The listing builds one solid part. Answer for the finished solid, in the listing's coordinates (mm). A direction names the side the tool comes from. Coordinates: 2 decimals unless noted, no trailing zeros. Write each loop counter-clockwise with the first axis right and the second up, starting at its lowest first coordinate (ties: lowest second). Pieces come first, ordered by that corner, then holes. Notation, with made-up numbers: M -35,-2.5 L 18,-2.5 A15 cw 18,2.5 Z; hole C 33,36 d9. An arc over 180 degrees is marked long. Answer as CSV lines item,"result".
```python
from build123d import *

# Parameters (mm, degrees)
BOSS_EXTRUDE1_DEPTH = 3
SKETCH5_W           = 35
SKETCH5_H           = 23
BOSS_EXTRUDE2_DEPTH = 3
BOSS_EXTRUDE5_DEPTH = 35
BOSS_EXTRUDE8_START = -35
BOSS_EXTRUDE8_DEPTH = 35
CUT_EXTRUDE1_START  = -96
SKETCH11_R          = 2.9
CUT_EXTRUDE1_DEPTH  = 96
BOSS_EXTRUDE7_DEPTH = 1
SKETCH17_R          = 2.5
CUT_EXTRUDE2_DEPTH  = 10
SKETCH18_R          = 2
CUT_EXTRUDE3_DEPTH  = 10
SKETCH19_R          = 2
CUT_EXTRUDE4_DEPTH  = 4
SKETCH21_R          = 2
CUT_EXTRUDE5_DEPTH  = 7
SKETCH22_R          = 2.5
CUT_EXTRUDE6_DEPTH  = 4
FILLET1_R           = 10
FILLET2_R           = 2
FILLET3_R           = 2
FILLET4_R           = 1


with BuildPart() as part:
    # Sketch1 → Boss-Extrude1 (new body)
    with BuildSketch(Plane(origin=(0, 0, 0), x_dir=(1, 0, 0), z_dir=(0, 1, 0))):
        Polygon((0, 0), (0, 23), (8.5, 23), (8.5, 33), (17.5, 33), (17.5, 23), (26, 23), (26, 0), (61, 0), (61, 28.801365462), (61, 67.406151765), (50.5, 93.029580251), (50.5, 160), (-24.5, 160), (-24.5, 93.029580251), (-35, 67.406151765), (-35, 28.801365462), (-35, 0), align=None)
    extrude(amount=BOSS_EXTRUDE1_DEPTH)

    # Sketch5 → Boss-Extrude2 (add)
    with BuildSketch(Plane(origin=(0, 3, 0), x_dir=(1, 0, 0), z_dir=(0, 1, 0))):
        with Locations((-17.5, 11.5)):
            Rectangle(SKETCH5_W, SKETCH5_H)
        with Locations((43.5, 11.5)):
            Rectangle(SKETCH5_W, SKETCH5_H)
    extrude(amount=BOSS_EXTRUDE2_DEPTH)

    # Sketch12 → Boss-Extrude5 (add)
    with BuildSketch(Plane.ZY.offset(35)):
        with BuildLine():
            Line((-7.857598958, 0), (1.361945499, 0))
            ThreePointArc((1.361945499, 0), (-3.247826729, 8.5), (-7.857598958, 0))
        make_face()
    extrude(amount=-BOSS_EXTRUDE5_DEPTH)

    # Sketch15 → Boss-Extrude8 (add)
    with BuildSketch(Plane(origin=(61, 0, 0), x_dir=(0, 0, -1), z_dir=(1, 0, 0)).offset(BOSS_EXTRUDE8_START)):
        with BuildLine():
            Line((7.857598958, 0), (-1.361945499, 0))
            ThreePointArc((-1.361945499, 0), (3.247826729, 8.5), (7.857598958, 0))
        make_face()
    extrude(amount=BOSS_EXTRUDE8_DEPTH)

    # Sketch11 → Cut-Extrude1 (cut)
    with BuildSketch(Plane.ZY.offset(35).offset(CUT_EXTRUDE1_START)):
        with Locations((-3.247826729, 3)):
            Circle(SKETCH11_R)
    extrude(amount=CUT_EXTRUDE1_DEPTH, mode=Mode.SUBTRACT)

    # Sketch14 → Boss-Extrude7 (add)
    with BuildSketch(Plane.XZ):
        Polygon((50.5, -93.029580251), (61, -67.406151765), (61, 1.361945499), (26, 1.361945499), (26, -23), (17.5, -23), (17.5, -33), (8.5, -33), (8.5, -23), (0, -23), (0, 1.361945499), (-35, 1.361945499), (-35, -67.406151765), (-24.5, -93.029580251), (-24.5, -160), (50.5, -160), align=None)
    extrude(amount=BOSS_EXTRUDE7_DEPTH)

    # Sketch17 → Cut-Extrude2 (cut)
    with BuildSketch(Plane(origin=(0, 3, 0), x_dir=(1, 0, 0), z_dir=(0, 1, 0))):
        with Locations(Location((-24.5, 33, 0), (0, 0, 270))):
            Circle(SKETCH17_R)
        with Locations(Location((50.5, 33, 0), (0, 0, 270))):
            Circle(SKETCH17_R)
    extrude(amount=-CUT_EXTRUDE2_DEPTH, mode=Mode.SUBTRACT)

    # Sketch18 → Cut-Extrude3 (cut)
    with BuildSketch(Plane(origin=(0, 3, 0), x_dir=(1, 0, 0), z_dir=(0, 1, 0))):
        with Locations(Location((-6.941705, 148.716738, 0), (0, 0, 270))):
            Circle(SKETCH18_R)
        with Locations(Location((32.941705, 148.716738, 0), (0, 0, 90))):
            Circle(SKETCH18_R)
    extrude(amount=-CUT_EXTRUDE3_DEPTH, mode=Mode.SUBTRACT)

    # Sketch19 → Cut-Extrude4 (cut)
    with BuildSketch(Plane(origin=(0, 3, 0), x_dir=(1, 0, 0), z_dir=(0, 1, 0))):
        with Locations(Location((-12.17438, 120.25, 0), (0, 0, 270))):
            Circle(SKETCH19_R)
        with Locations(Location((2.57562, 135, 0), (0, 0, 90))):
            Circle(SKETCH19_R)
        with Locations(Location((24.49992, 42, 0), (0, 0, 270))):
            Circle(SKETCH19_R)
        with Locations(Location((38.99992, 56.5, 0), (0, 0, 90))):
            Circle(SKETCH19_R)
    extrude(amount=-CUT_EXTRUDE4_DEPTH, mode=Mode.SUBTRACT)

    # Sketch21 → Cut-Extrude5 (cut)
    with BuildSketch(Plane(origin=(0, 6, 0), x_dir=(1, 0, 0), z_dir=(0, 1, 0))):
        with Locations(Location((-13.8, 18.7451, 0), (0, 0, 270))):
            Circle(SKETCH21_R)
        with Locations(Location((2.6, 30.245, 0), (0, 0, 270))):
            Circle(SKETCH21_R)
        with Locations(Location((23.4, 30.245, 0), (0, 0, 270))):
            Circle(SKETCH21_R)
        with Locations(Location((39.8, 18.7451, 0), (0, 0, 90))):
            Circle(SKETCH21_R)
    extrude(amount=-CUT_EXTRUDE5_DEPTH, mode=Mode.SUBTRACT)

    # Sketch22 → Cut-Extrude6 (cut)
    with BuildSketch(Plane(origin=(0, 3, 0), x_dir=(1, 0, 0), z_dir=(0, 1, 0))):
        with Locations(Location((-19, 133, 0), (0, 0, 270))):
            Circle(SKETCH22_R)
        with Locations(Location((45, 133, 0), (0, 0, 90))):
            Circle(SKETCH22_R)
    extrude(amount=-CUT_EXTRUDE6_DEPTH, mode=Mode.SUBTRACT)

    # Fillet1
    fillet1_edges = [part.edges().sort_by_distance(p)[0] for p in [
        (-24.5, 1, -160),
        (50.5, 1, -160),
    ]]
    fillet(fillet1_edges, radius=FILLET1_R)

    # Fillet2
    fillet2_edges = [part.edges().sort_by_distance(p)[0] for p in [
        (50.5, 1, -93.029580251),
        (61, 1, -67.406151765),
        (-17.5, 3, -23),
        (43.5, 3, -23),
        (-17.5, 6, -7.857598958),
        (43.5, 6, -7.857598958),
    ]]
    fillet(fillet2_edges, radius=FILLET2_R)

    # Fillet3
    fillet3_edges = [part.edges().sort_by_distance(p)[0] for p in [
        (-35, 1, -67.406151765),
        (-24.5, 1, -93.029580251),
    ]]
    fillet(fillet3_edges, radius=FILLET3_R)

    # Fillet4
    fillet4_edges = [part.edges().sort_by_distance(p)[0] for p in [
        (26, 1, -23),
        (17.5, 1, -23),
        (17.5, 1, -33),
        (8.5, 1, -33),
        (8.5, 1, -23),
        (0, 1, -23),
    ]]
    fillet(fillet4_edges, radius=FILLET4_R)


solid = part.part
```
Q1. Find section A-A (z = -12). Give the vertices of the cut face in (x, y).
Output:
outline,"M -35,-1 L 0,-1 L 0,6 L -35,6 Z; M 26,-1 L 61,-1 L 61,6 L 26,6 Z"
Q2. Flat-ended cylindrical pins translate along their axes: pin 1 Ø5 at (x, y) = (37.5, 6) entering from -Z; pin 2 Ø4 at (x, z) = (42.5, -14) entering from +Y; pin 3 Ø4.5 at (x, y) = (5.5, 1.5) entering from +Z. Find the tip coordinate at first contact, or state that the pin passes through.
Output:
pin 1,"z = -23.68"
pin 2,"y = 6"
pin 3,"z = -23"
Q3. For faces 5 (the flat face through (-18, 6, -16)), 6 (the cylindrical face through (-12.09, 1.03, -122.25)), 7 (the flat face through (4, 1, -23)), determine the directions among +Z, -Z, +X, -X, +Y, -Y from which every point of the face is accessible in a straight line to the end or side of a thin tool.
Output:
face 5,"-Z, +X, -X, +Y"
face 6,"+Y, -Y"
face 7,"+Z, +Y, -Y"
Q4. The mould has two halves that part along X. Classify faces 1 (the flat face through (17.5, 1, -28)), 2 (the cylindrical face through (-7.71, 1.03, -146.87)), 3 (the cylindrical face through (-17.745, 7.296, 0.186)), 4 (the flat face through (61, 2, -33)): pulls with the +X half, pulls with the -X half, needs draft (parallel to the pull), parting line crosses it, or undercut.
Output:
face 1,"undercut"
face 2,"undercut"
face 3,"needs draft"
face 4,"pulls with the +X half"
Q5. Straight lines are drawn through the part: line 1 (Z direction, x = 39.8, y = 2.5); line 2 (Z direction, x = 38.5, y = 2.25); line 3 (X direction, y = 2.25, z = -12). For each, find the intervals that lie inside material, in ascending order.
Output:
line 1,"-160 to -58.33, -54.67 to -20.75, -16.75 to -6.1, -0.39 to 2.23"
line 2,"-160 to -58.44, -54.56 to -20.26, -17.23 to -6.05, -0.45 to 2.2"
line 3,"-35 to 0, 26 to 61"
Q6. Find section C-C (z = -120.25). Give the vertices of the cut face in (x, y).
Output:
outline,"M -24.5,-1 L -14.17,-1 L -14.17,3 L -24.5,3 Z; M -10.17,-1 L 50.5,-1 L 50.5,3 L -10.17,3 Z"
Q7. Find section D-D (x = 13.5). Give the vertices of the cut face in (y, z), and give its area (3 significant figures).
Output:
outline,"M -1,-160 L 3,-160 L 3,-33 L -1,-33 Z"
area,"508 mm2"
Q8. Find section B-B (x = -2.5). Give the vertices of the cut face in (y, z).
Output:
outline,"M -1,-160 L 3,-160 L 3,-25 A2 cw 5,-23 L 6,-23 L 6,-8.84 A2 cw 6.67,-7.35 A5.5 ccw 0,1.36 L -1,1.36 Z; hole C 3,-3.25 d5.8"
